The listing builds one solid part. Answer for the finished solid, in the listing's coordinates (mm). A direction names the side the tool comes from. Give positions to 0.01 mm unless a question says otherwise; leave off trailing zeros. Order: outer loops, then holes, each group sorted by start corner. A loop starts at its lowest first (then second) coordinate and runs counter-clockwise, first axis right, second up. Notation, with made-up numbers: M -25.5,22 L -0.5,22 A24 cw -0.5,55 Z; hole C 81,89 d2. An arc over 180 degrees is marked long. Answer as a JSON object with one key per item and string values. Group by question number.
```python
from build123d import *

# Parameters (mm, degrees)
PAD_DEPTH    = 20
POCKET_DEPTH = 10


with BuildPart() as part:
    # Sketch → Pad (new body)
    with BuildSketch(Plane.XZ):
        with BuildLine():
            ThreePointArc((0, 0), (5.749809, -11.188952), (17.230824, -16.330866))
            ThreePointArc((17.230824, -16.330866), (105, -20), (192.769176, -16.330866))
            ThreePointArc((192.769176, -16.330866), (204.250191, -11.188952), (210, 0))
            ThreePointArc((210, 0), (211.364147, 40.039591), (204.5, 79.51))
            ThreePointArc((204.5, 79.51), (200.133385, 86.009194), (192.769176, 88.669134))
            ThreePointArc((192.769176, 88.669134), (105, 90), (17.230824, 88.669134))
            ThreePointArc((17.230824, 88.669134), (9.866615, 86.009194), (5.5, 79.51))
            ThreePointArc((5.5, 79.51), (-1.364147, 40.039591), (0, 0))
        make_face()
    extrude(amount=PAD_DEPTH)

    # Sketch001 (on Face10 of Pad) → Pocket (cut)
    with BuildSketch(Plane.XZ.offset(20)):
        with BuildLine():
            ThreePointArc((164.624157, 80.885897), (105, 83.1), (45.375843, 80.885897))
            ThreePointArc((45.375843, 80.885897), (40.44004, 77.994973), (39.7, 72.322942))
            Line((39.7, 72.322942), (55.5, 25.565661))
            ThreePointArc((55.5, 25.565661), (60.452364, 18.259103), (68.455126, 14.535192))
            ThreePointArc((68.455126, 14.535192), (105, 11.5), (141.544874, 14.535192))
            ThreePointArc((141.544874, 14.535192), (149.547636, 18.259103), (154.5, 25.565661))
            Line((170.3, 72.322942), (154.5, 25.565661))
            ThreePointArc((170.3, 72.322942), (169.55996, 77.994973), (164.624157, 80.885897))
        make_face()
    extrude(amount=-POCKET_DEPTH, mode=Mode.SUBTRACT)


solid = part.part
```
Item 1: Determine the mould class of faces 1 (the flat face through (162.51, -15.07, 49.27)), 2 (the cylindrical face through (204.12, -9.86, -11.31)), 3 (the cylindrical face through (104, -10, -20)), 4 (the cylindrical face through (-1.325, -9.86, 40.6)) for opening direction X: released by +X, released by -X, zero draft, split by the parting line, or undercut.
Item 2: Section C-C (z = 30) is taken. Determine the outline of the cut face in (x, y), and give its area (3 significant figures).
Item 3: A tool of negligible diameter and unlimited length cuts with its end or side. For faces 5 (the cylindrical face through (106, -10, 90)), 6 (the cylindrical face through (200.22, -9.86, 85.94)), 7 (the cylindrical face through (105.8, -15.1, 83.1)), from which of +Z, -Z, +X, -X, +Y, -Y can it reach the whole face along a straight path? Write none if from no direction.
Item 4: Section B-B (y = -3.5) is taken. Determine the outline of the cut face in (x, z).
Item 5: Section A-A (y = -17) is taken. Determine the outline of the cut face in (x, z).
Item 6: Consider probe 1 along Y at (x, z) = (158.5, 48.5); probe 2 along X at (y, z) = (-15.5, 22); probe 3 along X at (y, z) = (-11.25, 36). Determine where each line is inside the solid, lowest interval first. Write a range as from..to.
Item 7: Section D-D (x = 11) is taken. Determine the outline of the cut face in (y, z).
Item 8: Flat-ended cylindrical pins translate along their axes: P1, Ø12, axis at y = -10, z = 56, coming from the -X side; P2, Ø5, axis at x = 137.5, y = -10.5, coming from the +Z side; P3, Ø2, axis at x = 97.5, z = 31, coming from the -Y side. Find the tip coordinate at first contact, or state that the pin passes through.
Values found:
{
 "1": {"face 1": "undercut", "face 2": "released by +X", "face 3": "split by the parting line", "face 4": "released by -X"},
 "2": {"outline": "M -1.8,-20 L 54,-20 L 54,-10 L 156,-10 L 156,-20 L 211.8,-20 L 211.8,0 L -1.8,0 Z", "area": "3,250 mm^2"},
 "3": {"face 5": "+Z, +Y, -Y", "face 6": "+Z, +X, +Y, -Y", "face 7": "-Y"},
 "4": {"outline": "M 0,0 A18.99 ccw 17.23,-16.33 A1051.6 ccw 192.77,-16.33 A18.99 ccw 210,0 A194.6 ccw 204.5,79.51 A12.59 ccw 192.77,88.67 A2894.81 ccw 17.23,88.67 A12.59 ccw 5.5,79.51 A194.6 ccw Z"},
 "5": {"outline": "M 0,0 A18.99 ccw 17.23,-16.33 A1051.6 ccw 192.77,-16.33 A18.99 ccw 210,0 A194.6 ccw 204.5,79.51 A12.59 ccw 192.77,88.67 A2894.81 ccw 17.23,88.67 A12.59 ccw 5.5,79.51 A194.6 ccw Z; hole M 39.7,72.32 L 55.5,25.57 A16.56 ccw 68.46,14.54 A221.52 ccw 141.54,14.54 A16.56 ccw 154.5,25.57 L 170.3,72.32 A6.5 ccw 164.62,80.89 A803.92 ccw 45.38,80.89 A6.5 ccw Z"},
 "6": {"probe 1": "y = -10..0", "probe 2": "x = -1.77..57.2, 152.8..211.77", "probe 3": "x = -1.6..51.97, 158.03..211.6"},
 "7": {"outline": "M -20,-14.71 L 0,-14.71 L 0,86.8 L -20,86.8 Z"},
 "8": {"P1": "stops at x = -0.42", "P2": "stops at z = 89.84", "P3": "stops at y = -10"}
}
